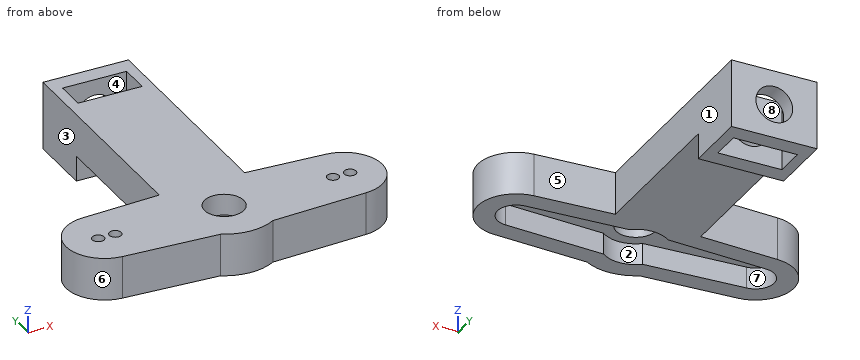
Autodesk Inventor part; units mm, degrees
ref_plane "Work Plane1" through (-16.55, 6.25, 30.8) normal (0, 0, 1) x (-1, 0, 0)
ref_plane "Work Plane2" through (0, 14.75, 0) normal (0, 1, 0) x (-1, 0, 0)
ref_plane "YZ Plane" through (0, 0, 0) normal (1, 0, 0) x (0, 1, 0)
ref_plane "Work Plane1" through (-16.55, 6.25, 30.8) normal (0, 0, 1) x (-1, 0, 0)
sketch "Sketch1" plane through (-16.55, 6.25, 30.8) normal (0, 0, 1) x (-1, 0, 0)
  circle A0 centre (4.7413, 0) radius 0.35
  circle A1 centre (6.7413, 0) radius 0.35
  circle A2 centre (8.7413, 0) radius 0.35
  circle A3 centre (10.7413, 0) radius 0.35
  circle A4 centre (12.7413, 0) radius 0.35
  circle A5 centre (14.7413, 0) radius 0.35
  circle A6 centre (-4.7413, 0) radius 0.35
  circle A7 centre (-6.7413, 0) radius 0.35
  circle A8 centre (-8.7413, 0) radius 0.35
  circle A9 centre (-10.7413, 0) radius 0.35
  circle A10 centre (-12.7413, 0) radius 0.35
  circle A11 centre (-14.7413, 0) radius 0.35
  circle A12 centre (0, 0) radius 2.3
  line L0 (2.2091, 2.65) -> (14.1096, 1.997)
  arc A13 (2.2091, 2.65) -> (-2.2091, 2.65) centre (0, 0) ccw
  line L1 (-14.1096, 1.997) -> (-2.2091, 2.65)
  arc A14 (-14.1096, 1.997) -> (-14.1096, -1.997) centre (-14, 0) ccw
  line L2 (-2.2091, -2.65) -> (-14.1096, -1.997)
  arc A15 (-2.2091, -2.65) -> (2.2091, -2.65) centre (0, 0) ccw
  line L3 (14.1096, -1.997) -> (2.2091, -2.65)
  arc A16 (14.1096, -1.997) -> (14.1096, 1.997) centre (14, 0) ccw
  arc A17 (2.2852, 2.8461) -> (-2.2852, 2.8461) centre (0, 0) ccw
  line L4 (2.2852, 2.8461) -> (14.1205, 2.1967)
  arc A18 (14.1205, -2.1967) -> (14.1205, 2.1967) centre (14, 0) ccw
  line L5 (14.1205, -2.1967) -> (2.2852, -2.8461)
  arc A19 (-2.2852, -2.8461) -> (2.2852, -2.8461) centre (0, 0) ccw
  line L6 (-2.2852, -2.8461) -> (-14.1205, -2.1967)
  arc A20 (-14.1205, 2.1967) -> (-14.1205, -2.1967) centre (-14, 0) ccw
  line L7 (-14.1205, 2.1967) -> (-2.2852, 2.8461)
  arc A21 (3.0522, 5.1075) -> (-3.0522, 5.1075) centre (0, 0) ccw
  line L8 (3.0522, 5.1075) -> (14.2466, 4.4932)
  arc A22 (14.2466, -4.4932) -> (14.2466, 4.4932) centre (14, 0) ccw
  line L9 (14.2466, -4.4932) -> (3.0522, -5.1075)
  arc A23 (-3.0522, -5.1075) -> (3.0522, -5.1075) centre (0, 0) ccw
  line L10 (-3.0522, -5.1075) -> (-14.2466, -4.4932)
  arc A24 (-14.2466, 4.4932) -> (-14.2466, -4.4932) centre (-14, 0) ccw
  line L11 (-14.2466, 4.4932) -> (-3.0522, 5.1075)
  circle A25 centre (-14.7413, 0) radius 0.35
  point P0 (-16.55, 6.25)
  dimension "d0" = 0.2
  dimension "d1" = 2.5
extrude "Extrusion1" add sketch "Sketch1" against normal blind 2.5 contours L8 A22 L9 A23 L10 A24 L11 A21
sketch "Sketch2" plane through (-16.55, 6.25, 30.8) normal (0, 0, 1) x (1, 0, 0)
  arc A0 (-3.0522, -5.1075) -> (3.0522, -5.1075) centre (0, 0) ccw
  line L0 (14.2466, -4.4932) -> (3.0522, -5.1075)
  arc A1 (14.2466, -4.4932) -> (14.2466, 4.4932) centre (14, 0) ccw
  line L1 (3.0522, 5.1075) -> (14.2466, 4.4932)
  arc A2 (3.0522, 5.1075) -> (-3.0522, 5.1075) centre (0, 0) ccw
  line L2 (-14.2466, 4.4932) -> (-3.0522, 5.1075)
  arc A3 (-14.2466, 4.4932) -> (-14.2466, -4.4932) centre (-14, 0) ccw
  line L3 (-3.0522, -5.1075) -> (-14.2466, -4.4932)
  line L4 (14.1205, -2.1967) -> (2.2852, -2.8461)
  arc A4 (-2.2852, -2.8461) -> (2.2852, -2.8461) centre (0, 0) ccw
  line L5 (-2.2852, -2.8461) -> (-14.1205, -2.1967)
  arc A5 (-14.1205, 2.1967) -> (-14.1205, -2.1967) centre (-14, 0) ccw
  line L6 (-14.1205, 2.1967) -> (-2.2852, 2.8461)
  arc A6 (2.2852, 2.8461) -> (-2.2852, 2.8461) centre (0, 0) ccw
  line L7 (2.2852, 2.8461) -> (14.1205, 2.1967)
  arc A7 (14.1205, -2.1967) -> (14.1205, 2.1967) centre (14, 0) ccw
  arc A8 (-3.0522, -5.1075) -> (3.0522, -5.1075) centre (0, 0) ccw
  line L8 (14.2466, -4.4932) -> (3.0522, -5.1075)
  arc A9 (14.2466, -4.4932) -> (14.2466, 4.4932) centre (14, 0) ccw
  line L9 (3.0522, 5.1075) -> (14.2466, 4.4932)
  arc A10 (3.0522, 5.1075) -> (-3.0522, 5.1075) centre (0, 0) ccw
  line L10 (-14.2466, 4.4932) -> (-3.0522, 5.1075)
  arc A11 (-14.2466, 4.4932) -> (-14.2466, -4.4932) centre (-14, 0) ccw
  line L11 (-3.0522, -5.1075) -> (-14.2466, -4.4932)
  circle A12 centre (-14.7413, 0) radius 0.35
  circle A13 centre (-12.7413, 0) radius 0.35
  circle A14 centre (12.7413, 0) radius 0.35
  circle A15 centre (14.7413, 0) radius 0.35
  circle A16 centre (0, 0) radius 2.3
  point P0 (16.55, -6.25)
extrude "Extrusion2" add sketch "Sketch2" along normal blind 2.5 contours L3 A3 L2 A2 L1 A1 L0 A0 | L4 A4 L5 A5 L6 A6 L7 A7
sketch "Sketch3" plane through (-16.55, 6.25, 33.3) normal (0, 0, 1) x (1, 0, 0)
  circle A0 centre (14.7413, 0) radius 0.35
  circle A1 centre (12.7413, 0) radius 0.35
  circle A2 centre (-12.7413, 0) radius 0.35
  circle A3 centre (-14.7413, 0) radius 0.35
  circle A4 centre (-14.7413, 0) radius 0.7
  circle A5 centre (-12.7413, 0) radius 0.7
  circle A6 centre (12.7413, 0) radius 0.7
  circle A7 centre (14.7413, 0) radius 0.7
  point P0 (16.55, -6.25)
  dimension "d6" = 1.4
  dimension "d7" = 1.4
  dimension "d8" = 1.4
  dimension "d9" = 1.4
extrude "Extrusion3" cut sketch "Sketch3" against normal up to next
ref_plane "Work Plane2" through (0, 14.75, 0) normal (0, 1, 0) x (-1, 0, 0)
sketch "Sketch4" plane through (0, 14.75, 0) normal (0, 1, 0) x (-1, 0, 0)
  line L0 (19.6022, 33.3) -> (30.7966, 33.3) construction
  line L1 (30.7966, 28.3) -> (19.6022, 28.3) construction
  line L2 (2.3034, 33.3) -> (13.4978, 33.3) construction
  line L3 (13.4978, 28.3) -> (2.3034, 28.3) construction
  line L4 (11.55, 33.3) -> (21.55, 33.3)
  line L5 (21.55, 33.3) -> (21.55, 28.3)
  line L6 (21.55, 28.3) -> (11.55, 28.3)
  line L7 (11.55, 28.3) -> (11.55, 33.3)
  line L8 (-1.95, 33.3) -> (-1.95, 28.3) construction
  line L9 (35.05, 33.3) -> (35.05, 28.3) construction
  point P0 (0, 0)
  dimension "d13" = 10
  dimension "d14" = 13.5
extrude "Extrusion4" add sketch "Sketch4" against normal up to next
sketch "Sketch5" plane through (0, 14.75, 0) normal (0, 1, 0) x (1, 0, 0)
  line L0 (-11.55, -33.3) -> (-21.55, -33.3)
  line L1 (-11.55, -28.3) -> (-11.55, -33.3)
  line L2 (-21.55, -28.3) -> (-11.55, -28.3)
  line L3 (-21.55, -33.3) -> (-21.55, -28.3)
  point P0 (0, 0)
extrude "Extrusion5" add sketch "Sketch5" along normal blind 22.7
sketch "Sketch6" plane through (-16.55, 6.25, 28.3) normal (0, 0, -1) x (-1, 0, 0)
  line L0 (-5, 31.2) -> (5, 31.2)
  line L1 (-5, 31.2) -> (-5, 5.0006)
  line L2 (-3.75, 29.2) -> (3.75, 29.2)
  line L3 (3.75, 29.2) -> (3.75, 25.7)
  line L4 (3.75, 25.7) -> (-3.75, 25.7)
  line L5 (-3.75, 25.7) -> (-3.75, 29.2)
  point P0 (-16.55, -6.25)
  dimension "d19" = 7.5
  dimension "d20" = 3.5
  dimension "d21" = 1.25
  dimension "d22" = 2
extrude "Extrusion6" cut sketch "Sketch6" against normal up to next
sketch "Sketch7" plane through (-16.55, 6.25, 28.3) normal (0, 0, -1) x (-1, 0, 0)
  line L0 (-3.75, 25.7) -> (-3.75, 29.2)
  line L1 (-3.75, 29.2) -> (3.75, 29.2)
  line L2 (3.75, 29.2) -> (3.75, 25.7)
  line L3 (3.75, 25.7) -> (-3.75, 25.7)
  line L4 (5, 31.2) -> (5, 5.0006)
  line L5 (-5, 31.2) -> (5, 31.2)
  line L6 (5, 31.2) -> (5, 23.7)
  line L7 (5, 23.7) -> (-5, 23.7)
  line L8 (-5, 23.7) -> (-5, 31.2)
  point P0 (-16.55, -6.25)
  dimension "d25" = 7.5
extrude "Extrusion7" add sketch "Sketch7" along normal blind 3
sketch "Sketch8" plane through (0, 37.45, 0) normal (0, 1, 0) x (1, 0, 0)
  circle A0 centre (-16.55, -29.3) radius 2.15
  point P0 (0, 0)
  dimension "d28" = 4.3
extrude "Extrusion8" cut sketch "Sketch8" against normal blind 11
properties part number "HornPocket"
The listing builds one solid part. Answer for the finished solid, in the listing's coordinates (mm). Face numbers are marked on the shaded views. A direction names the side the tool comes from. Coordinates: 2 decimals unless noted, no trailing zeros. Loops run counter-clockwise (first coordinate to the right, second up) from the corner with the lowest first, then second, coordinate; pieces in that order, holes last. Notation, with made-up numbers: M 53.5,28.25 L 99.5,28.25 A13 ccw 99.5,36.25 Z; hole C -23.75,76 d3. An arc over 180 degrees is marked long. Answer as a JSON object with one key per item and string values. Group by question number.
Item 1: Section A-A (x = -16.55) is taken. Write down the section's boundary in (y, z).
Item 2: Which of the six approach directions +Z, -Z, +X, -X, +Y, -Y give full straight-line access (tool end or side, diameter ignored) to the marked faces 1, 2, 3 and 4?
Item 3: Each of these flat-tipped pins is pushed along its axis until it touches: P1, Ø4, axis at x = -16.55, z = 29.3, coming from the +Y side; P2, Ø8, axis at x = -17, y = 13, coming from the -Z side; P3, Ø1.5, axis at x = -9.5, z = 27.5, coming from the +Y side; P4, Ø4, axis at y = 33, z = 31, coming from the -X side. Where does it stop, or does it pass through?
Item 4: Section D-D (z = 32.75) is taken. Write down the section's boundary in (x, y).
Item 5: Consider L1, parallel to Y at x = -16.5, z = 32; L2, parallel to X at y = 29.7, z = 29.3; L3, parallel to X at y = 32.5, z = 25.5. Determine where each line is inside the solid, lowest interval first.
Item 6: Determine the mould class of the marked faces 5, 6, 7 and 8 for opening direction X: +X half, -X half, draft (parallel to the pull), parting line (faces both ways), or undercut.
Item 7: Section B-B (y = 6.25) is taken. Write down the section's boundary in (x, z).
Solved:
{
 "1": {"outline": "M 0.3,28.3 L 2.6,28.3 L 2.6,30.8 L 3.95,30.8 L 3.95,33.3 L 0.3,33.3 Z; M 8.55,30.8 L 9.9,30.8 L 9.9,28.3 L 26.45,28.3 L 26.45,31.45 L 31.95,31.45 L 31.95,33.3 L 8.55,33.3 Z; M 29.95,25.3 L 31.95,25.3 L 31.95,27.15 L 29.95,27.15 Z; M 35.45,25.3 L 37.45,25.3 L 37.45,27.15 L 35.45,27.15 Z; M 35.45,31.45 L 37.45,31.45 L 37.45,33.3 L 35.45,33.3 Z"},
 "2": {"face 1": "+Z, -Z, +X, +Y", "face 2": "-Z", "face 3": "+Z, -Z, -X, +Y", "face 4": "+Z, -Z"},
 "3": {"P1": "stops at y = 26.45", "P2": "stops at z = 28.3", "P3": "passes through", "P4": "stops at x = -21.55"},
 "4": {"outline": "M -30.8,1.76 L -19.6,1.14 A5.95 ccw -13.5,1.14 L -2.3,1.76 A4.5 ccw -2.3,10.74 L -11.55,11.25 L -11.55,37.45 L -21.55,37.45 L -21.55,11.25 L -30.8,10.74 A4.5 ccw Z; hole C -31.29,6.25 d1.4; hole C -29.29,6.25 d1.4; hole M -20.3,31.95 L -12.8,31.95 L -12.8,35.45 L -20.3,35.45 Z; hole C -16.55,6.25 d4.6; hole C -3.81,6.25 d1.4; hole C -1.81,6.25 d1.4"},
 "5": {"L1": "y = 0.3 to 3.95, 8.55 to 31.95, 35.45 to 37.45", "L2": "x = -21.55 to -18.7, -14.4 to -11.55", "L3": "x = -21.55 to -20.3, -12.8 to -11.55"},
 "6": {"face 5": "+X half", "face 6": "-X half", "face 7": "undercut", "face 8": "undercut"},
 "7": {"outline": "M -35.05,28.3 L -32.75,28.3 L -32.75,30.8 L -31.99,30.8 L -31.99,33.3 L -35.05,33.3 Z; M -30.59,30.8 L -29.99,30.8 L -29.99,33.3 L -30.59,33.3 Z; M -28.59,30.8 L -18.85,30.8 L -18.85,33.3 L -28.59,33.3 Z; M -14.25,30.8 L -4.51,30.8 L -4.51,33.3 L -14.25,33.3 Z; M -3.11,30.8 L -2.51,30.8 L -2.51,33.3 L -3.11,33.3 Z; M -1.11,30.8 L -0.35,30.8 L -0.35,28.3 L 1.95,28.3 L 1.95,33.3 L -1.11,33.3 Z"}
}
